Autodesk Inventor part; units mm, degrees
ref_plane "YZ Plane" through (0, 0, 0) normal (1, 0, 0) x (0, 1, 0)
ref_plane "XZ Plane" through (0, 0, 0) normal (0, 1, 0) x (-1, 0, 0)
ref_plane "XY Plane" through (0, 0, 0) normal (0, 0, 1) x (1, 0, 0)
sketch "Szkic1" plane through (0, 0, 0) normal (0, 1, 0) x (-1, 0, 0)
  line L0 (34.3124, 12.606) -> (49, 12.606)
  line L1 (0, 12.606) -> (0, -21.394)
  line L2 (20, -21.394) -> (22.7076, -21.394)
  line L3 (49, 12.606) -> (32.75, 12.606)
  line L4 (32.3719, 11.09) -> (24.6481, -19.878)
  arc A0 (34.3124, 12.606) -> (32.3719, 11.09) centre (34.3124, 10.606) ccw
  arc A1 (22.7076, -21.394) -> (24.6481, -19.878) centre (22.7076, -19.394) ccw
  line L5 (49, 12.606) -> (49, 22.606)
  line L6 (49, 22.606) -> (0, 22.606)
  line L7 (0, 22.606) -> (0, 12.606)
  line L8 (0, -21.394) -> (18, -21.394)
  line L9 (18, -23.394) -> (18, -36.124)
  line L10 (18, -36.124) -> (0, -36.124)
  line L11 (0, -36.124) -> (0, -21.394)
  arc A2 (20, -21.394) -> (18, -23.394) centre (20, -23.394) ccw
  point P0 (0, 0)
  point P1 (24.27, -21.394)
  dimension "d0" = 49
  dimension "d1" = 34
  dimension "d2" = 24.27
  dimension "d3" = 16.25
  dimension "d4" = 2
  dimension "d5" = 2
  dimension "d6" = 10
  dimension "d7" = 18
  dimension "d8" = 14.73
  dimension "d9" = 2
revolve "Obrót1" add sketch "Szkic1" angle 360 about axis through (0, 0, 12.606) along (0, 0, -1)
sketch "Szkic4" plane through (0, 0, 22.606) normal (0, 0, 1) x (1, 0, 0)
  circle A0 centre (0, 0) radius 8
  dimension "d16" = 16
sketch "Szkic5" plane through (0, 0, 22.606) normal (0, 0, 1) x (1, 0, 0)
  circle A0 centre (0, 0) radius 40
  circle A1 centre (-40, 0) radius 4.5
  circle A2 centre (0, -40) radius 4.5
  circle A3 centre (40, 0) radius 4.5
  circle A4 centre (0, 40) radius 4.5
  point P0 (-39.7469, -4.4929)
  point P1 (-39.7469, 4.4929)
  dimension "d21" = 80
  dimension "d22" = 9
  dimension "d31" = 9
  dimension "d32" = 9
  dimension "d33" = 9
extrude "Wyciągnięcie proste3" cut sketch "Szkic5" against normal through all contours A0 A3 | A0 A3 | A4 A0 | A0 A4 | A2 A0 | A0 A2 | A1 A0 | A0 A1
extrude "Wyciągnięcie proste5" cut sketch "Szkic4" against normal blind 60
sketch "Szkic7" plane through (0, 0, 22.606) normal (0, 0, 1) x (1, 0, 0)
  circle A0 centre (0, 0) radius 29
extrude "Wyciągnięcie proste6" add sketch "Szkic7" along normal blind 12
sketch "Szkic8" plane through (0, 0, 34.606) normal (0, 0, 1) x (1, 0, 0)
  circle A0 centre (0, 0) radius 8
  circle A1 centre (0, 0) radius 20
extrude "Wyciągnięcie proste7" cut sketch "Szkic8" against normal blind 47 contours A0 | A1
sketch "Szkic9" plane through (0, 0, -12.394) normal (0, 0, 1) x (1, 0, 0)
  circle A0 centre (0, 0) radius 10
  circle A1 centre (0, 0) radius 8
extrude "Wyciągnięcie proste8" add sketch "Szkic9" along normal blind 7
properties part number "pokrywa" material "Srebro"
Can you work these out from the model? Positions are in its coordinate system, mm. A direction names the side the tool comes from. Coordinates: 2 decimals unless noted, no trailing zeros. Write each loop counter-clockwise with the first axis right and the second up, starting at its lowest first coordinate (ties: lowest second). Pieces come first, ordered by that corner, then holes. Notation, with made-up numbers: (-22, -18.75) -> (-7, -18.75) arc R6 ccw to (-7, -12.75) -> close; hole circle Ø11 at (-22, -34.5). An arc over 180 degrees is marked (long way). Answer as CSV lines item,"result".
1) If we section it at A-A on x = -40: Please give me the cut outline in (y, z).
Check result:
outline,"(-28.3, 12.61) -> (-4.5, 12.61) -> (-4.5, 22.61) -> (-28.3, 22.61) -> close; (4.5, 12.61) -> (28.3, 12.61) -> (28.3, 22.61) -> (4.5, 22.61) -> close"
2) Will these pins go through, and if not, where does the flat tip stop? P1, Ø10.5, axis at x = 0, y = -40, coming from the +Z side; P2, Ø3, axis at y = -37, z = 19.5, coming from the -X side (3 decimals); P3, Ø20, axis at x = 4.5, y = -3, coming from the +Z side.
Check result:
P1,"z = 22.61"
P2,"x = -33.775"
P3,"z = -5.39"
3) If I drill on line 1 (Y direction, x = 0, z = 18); line 2 (Y direction, x = 0, z = -26); line 3 (Y direction, x = 0, z = 11), over which ranges is the centre line in solid material (lowest first)? Write a range as from..to.
Check result:
line 1,"-49..-44.5, -35.5..-20, 20..35.5, 44.5..49"
line 2,"-18..-8, 8..18"
line 3,"-32.35..-20, 20..32.35"
4) If we section it at C-C on z = 20.5: Please give me the cut outline in (x, y).
Check result:
outline,"circle Ø98 at (0, 0); hole circle Ø9 at (-40, 0); hole circle Ø40 at (0, 0); hole circle Ø9 at (0, -40); hole circle Ø9 at (0, 40); hole circle Ø9 at (40, 0)"
5) If we mould it in two halves opening along Y, with no side actions, what happens to faces 4 (the flat face through (-21, -21, 22.606)), 5 (the cylindrical face through (-26.34, -41.32, 17.68)), 6 (the flat face through (0, 8.2, -5.394))? For each: +Y half, -Y half, draft (parallel to the pull), parting line (faces both ways), or undercut.
Check result:
face 4,"draft"
face 5,"parting line"
face 6,"undercut"
6) If we section it at B-B on y = -43: Please give me the cut outline in (x, z).
Check result:
outline,"(-23.49, 12.61) -> (-3.35, 12.61) -> (-3.35, 22.61) -> (-23.49, 22.61) -> close; (3.35, 12.61) -> (23.49, 12.61) -> (23.49, 22.61) -> (3.35, 22.61) -> close"
7) On a 3-axis mill with a long thin cutter (end or side, diameter ignored), from which of +Z, -Z, +X, -X, +Y, -Y can I reach the whole of each face in a straight line? I mean faces 1 (the cylindrical face through (44.292, 1.352, 17.676)), 2 (the flat face through (33, -11, 12.606)), 3 (the cylindrical face through (13.38, 25.73, 28.52)). Say none if no direction works.
Check result:
face 1,"+Z, -Z"
face 2,"-Z"
face 3,"+Z"
8) If we section it at D-D on x = 0: Count the separate pieces of the cut face and the enclosed holes in it, then the cut area to 4 significant figures.
Check result:
separate pieces,"4"
enclosed holes,"0"
area,"1,735 mm²"
